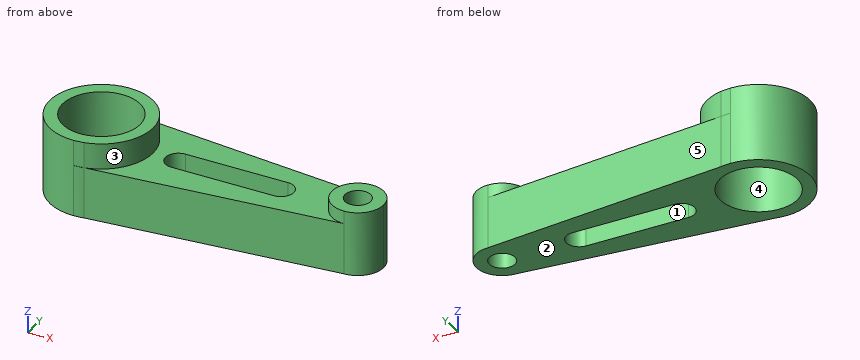
```python
from build123d import *

# Parameters (mm, degrees)
F0_R     = 19.05
F1_DEPTH = 25.4
F2_DEPTH = 38.1
F0_R_2   = 6.35
F3_DEPTH = 31.75


with BuildPart() as f1:
    # F0 (on Top) → F1 (new body)
    with BuildSketch(Plane.XY):
        with BuildLine():
            Line((-58.4702970297, 24.897029703), (-63.5, 25.4))
            ThreePointArc((-63.5, 25.4), (-88.9, 0), (-63.5, -25.4))
            Line((-63.5, -25.4), (-58.4702970297, -24.897029703))
            ThreePointArc((-58.4702970297, -24.897029703), (-43.8414846002, -16.0842398725), (-38.1, 0))
            ThreePointArc((-38.1, 0), (-43.8414846002, 16.0842398725), (-58.4702970297, 24.897029703))
        make_face()
        with Locations((-63.5, 0)):
            Circle(F0_R, mode=Mode.SUBTRACT)
        with BuildLine():
            ThreePointArc((-58.4702970297, 24.897029703), (-60.9726055369, 25.2739446313), (-63.5, 25.4))
            Line((-63.5, 25.4), (-58.4702970297, 24.897029703))
        make_face()
        with BuildLine():
            Line((-58.4702970297, -24.897029703), (-63.5, -25.4))
            ThreePointArc((-63.5, -25.4), (-60.9726055369, -25.2739446313), (-58.4702970297, -24.897029703))
        make_face()
        with BuildLine():
            Line((63.5, 12.7), (-58.4702970297, 24.897029703))
            ThreePointArc((-58.4702970297, 24.897029703), (-43.8414846002, 16.0842398725), (-38.1, 0))
            ThreePointArc((-38.1, 0), (-43.8414846002, -16.0842398725), (-58.4702970297, -24.897029703))
            Line((-58.4702970297, -24.897029703), (63.5, -12.7))
            ThreePointArc((63.5, -12.7), (50.8, 0), (63.5, 12.7))
        make_face()
        with BuildLine():
            ThreePointArc((-25.4, -6.35), (-31.75, 0), (-25.4, 6.35))
            Line((-25.4, 6.35), (25.4, 6.35))
            ThreePointArc((25.4, 6.35), (31.75, 0), (25.4, -6.35))
            Line((25.4, -6.35), (-25.4, -6.35))
        make_face(mode=Mode.SUBTRACT)
    extrude(amount=F1_DEPTH)

    # F0 (on Top) → F2 (join)
    with BuildSketch(Plane.XY):
        with BuildLine():
            Line((-58.4702970297, 24.897029703), (-63.5, 25.4))
            ThreePointArc((-63.5, 25.4), (-88.9, 0), (-63.5, -25.4))
            Line((-63.5, -25.4), (-58.4702970297, -24.897029703))
            ThreePointArc((-58.4702970297, -24.897029703), (-43.8414846002, -16.0842398725), (-38.1, 0))
            ThreePointArc((-38.1, 0), (-43.8414846002, 16.0842398725), (-58.4702970297, 24.897029703))
        make_face()
        with Locations((-63.5, 0)):
            Circle(F0_R, mode=Mode.SUBTRACT)
    extrude(amount=F2_DEPTH)

    # F0 (on Top) → F3 (join)
    with BuildSketch(Plane.XY):
        with BuildLine():
            ThreePointArc((76.2, 0), (72.4802561211, 8.9802561211), (63.5, 12.7))
            ThreePointArc((63.5, 12.7), (50.8, 0), (63.5, -12.7))
            ThreePointArc((63.5, -12.7), (72.4802561211, -8.9802561211), (76.2, 0))
        make_face()
        with Locations((63.5, 0)):
            Circle(F0_R_2, mode=Mode.SUBTRACT)
    extrude(amount=F3_DEPTH)


solid = f1.part
```
Here's how the part is built. I have some questions about the finished solid (model axes, mm). Face numbers are marked on the shaded views. A direction names the side the tool comes from. Coordinates: 2 decimals unless noted, no trailing zeros. Order: outer loops, then holes, each group sorted by start corner. A loop starts at its lowest first (then second) coordinate and runs counter-clockwise, first axis right, second up.
1) Will these pins go through, and if not, where does the flat tip stop? pin 1 (6 mm diameter, centred on y = 11, z = 25.5, fed in from +X); pin 2 (1.5 mm diameter, centred on x = 12.5, z = 5, fed in from +Y) (3 decimals); pin 3 (5 mm diameter, centred on x = 40, y = 15, fed in from +Z); pin 4 (20.5 mm diameter, centred on x = 63.5, y = 0, fed in from -Z).
2) We'd pull the mould along Y, two halves only. Please class the marked faces 3, 4 and 5: +Y half, -Y half, draft (parallel to the pull), parting line (faces both ways), or undercut.
3) Imagine slicing it at A-A on z = 11. List the corners of the cut face in (x, y) for me, and give its area (3 significant figures).
4) Imagine slicing it at D-D on y = 16.5. List the corners of the cut face in (x, z) for me.
5) Imagine slicing it at B-B on x = -55.5. List the corners of the cut face in (y, z) for me.
6) Imagine slicing it at C-C on y = 2. List the corners of the cut face in (x, z) for me.
7) I need wall thicknesses on line 1 (X direction, y = -0.5, z = 18.5); line 2 (Y direction, x = -63.5, z = 14.5); line 3 (Y direction, x = 63.5, z = 15.5). Which ranges of each line are inside material? Lowest first, please.
8) Which directions (+Z, -Z, +X, -X, +Y, -Y) give clear straight access to the entire face, cutting with the end or side of a thin tool? Please do the marked faces 1 and 2.
Response values:
1. pin 1: stops at x = 73.36
1. pin 2: stops at y = 17.875
1. pin 3: stops at z = 25.4
1. pin 4: stops at z = 0
2. face 3: parting line
2. face 4: undercut
2. face 5: +Y half
3. outline: (-58.47, -24.9) - (63.5, -12.7) arc R12.7 ccw to (63.5, 12.7) - (-58.47, 24.9) arc R25.4 ccw (long way) to start; hole circle Ø38.1 at (-63.5, 0); hole (-25.4, -6.35) - (25.4, -6.35) arc R6.35 ccw to (25.4, 6.35) - (-25.4, 6.35) arc R6.35 ccw to start; hole circle Ø12.7 at (63.5, 0)
3. area: 4,070 mm2
4. outline: (-82.81, 0) - (-73.02, 0) - (-73.02, 38.1) - (-82.81, 38.1) - close; (-53.98, 0) - (25.5, 0) - (25.5, 25.4) - (-44.19, 25.4) - (-44.19, 38.1) - (-53.98, 38.1) - close
5. outline: (-24.6, 0) - (-17.29, 0) - (-17.29, 38.1) - (-24.11, 38.1) - (-24.11, 25.4) - (-24.6, 25.4) - close; (17.29, 0) - (24.6, 0) - (24.6, 25.4) - (24.11, 25.4) - (24.11, 38.1) - (17.29, 38.1) - close
6. outline: (-88.82, 0) - (-82.44, 0) - (-82.44, 38.1) - (-88.82, 38.1) - close; (-44.56, 0) - (-31.43, 0) - (-31.43, 25.4) - (-38.18, 25.4) - (-38.18, 38.1) - (-44.56, 38.1) - close; (31.43, 0) - (57.47, 0) - (57.47, 31.75) - (50.96, 31.75) - (50.96, 25.4) - (31.43, 25.4) - close; (69.53, 0) - (76.04, 0) - (76.04, 31.75) - (69.53, 31.75) - close
7. line 1: x = -88.9 to -82.54, -44.46 to -31.73, 31.73 to 57.17, 69.83 to 76.19
7. line 2: y = -25.4 to -19.05, 19.05 to 25.4
7. line 3: y = -12.7 to -6.35, 6.35 to 12.7
8. face 1: +Z, -Z
8. face 2: -Z, +X, -X, +Y, -Y
